The model under review builds one solid part; all positions refer to its coordinate system, in mm. Round coordinates to 2 decimals unless told otherwise and drop trailing zeros. Write each loop counter-clockwise with the first axis right and the second up, starting at its lowest first coordinate (ties: lowest second). Pieces come first, ordered by that corner, then holes. Notation, with made-up numbers: (-5.5, 23) - (49.5, 23) arc R29 cw to (49.5, 49) - close; hole circle Ø10 at (17.5, 83). An arc over 180 degrees is marked (long way). Return JSON: item names as keys, results as strings.
from build123d import *

# Parameters (mm, degrees)
EXTRUDE001_DEPTH = 3
FACE001_W        = 6
FACE001_H        = 15.392872
EXTRUDE002_DEPTH = 3
EXTRUDE003_DEPTH = 3
FACE003_W        = 15.392872
FACE003_H        = 6
EXTRUDE004_DEPTH = 3
EXTRUDE005_DEPTH = 3
EXTRUDE006_DEPTH = 3
EXTRUDE007_DEPTH = 3
FACE007_W        = 10
FACE007_H        = 10
EXTRUDE008_DEPTH = 3
EXTRUDE009_DEPTH = 3
EXTRUDE010_DEPTH = 3
EXTRUDE012_DEPTH = 3
FACE012_W        = 6
FACE012_H        = 15.392872
EXTRUDE013_DEPTH = 3
FACE010_W        = 15.392872
FACE010_H        = 6
EXTRUDE011_DEPTH = 3
EXTRUDE_DEPTH    = 1.5


with BuildPart() as extrude001:
    # Face → Extrude001 (new body)
    with BuildSketch(Plane(origin=(-12.399665, 12.399665, 0), x_dir=(0, 1, 0), z_dir=(0, 0, 1))):
        Polygon((4, -2), (-2, 4), (-2, -2), align=None)
    extrude(amount=EXTRUDE001_DEPTH)


with BuildPart() as extrude002:
    # Face001 → Extrude002 (new body)
    with BuildSketch(Plane(origin=(0, 13.399665, 0), x_dir=(0, 1, 0), z_dir=(0, 0, 1))):
        Rectangle(FACE001_W, FACE001_H)
    extrude(amount=EXTRUDE002_DEPTH)


with BuildPart() as extrude003:
    # Face002 → Extrude003 (new body)
    with BuildSketch(Plane(origin=(12.399665, 12.399665, 0), x_dir=(0, 1, 0), z_dir=(0, 0, 1))):
        Polygon((-2, -4), (4, 2), (-2, 2), align=None)
    extrude(amount=EXTRUDE003_DEPTH)


with BuildPart() as extrude004:
    # Face003 → Extrude004 (new body)
    with BuildSketch(Plane(origin=(13.399665, 0, 0), x_dir=(0, 1, 0), z_dir=(0, 0, 1))):
        Rectangle(FACE003_W, FACE003_H)
    extrude(amount=EXTRUDE004_DEPTH)


with BuildPart() as extrude005:
    # Face004 → Extrude005 (new body)
    with BuildSketch(Plane(origin=(12.399665, -12.399665, 0), x_dir=(0, 1, 0), z_dir=(0, 0, 1))):
        Polygon((2, -4), (2, 2), (-4, 2), align=None)
    extrude(amount=EXTRUDE005_DEPTH)


with BuildPart() as extrude006:
    # Face005 → Extrude006 (new body)
    with BuildSketch(Plane(origin=(7.712675, 0, 0), x_dir=(0, -1, 0), z_dir=(0, 0, -1))):
        Polygon((5.998742, 0.712675), (-5.998742, 0.712675), (-6.697694, -0.686991), (6.697694, -0.686991), align=None)
    extrude(amount=-EXTRUDE006_DEPTH)


with BuildPart() as extrude007:
    # Face006 → Extrude007 (new body)
    with BuildSketch(Plane(origin=(0, 7.712675, 0), x_dir=(0, -1, 0), z_dir=(0, 0, -1))):
        Polygon((-0.686991, 6.697694), (-0.686991, -6.697694), (0.712675, -5.998742), (0.712675, 5.998742), align=None)
    extrude(amount=-EXTRUDE007_DEPTH)


with BuildPart() as extrude008:
    # Face007 → Extrude008 (new body)
    with BuildSketch(Plane(origin=(0, 0, 0), x_dir=(0, 1, 0), z_dir=(0, 0, 1))):
        Rectangle(FACE007_W, FACE007_H)
    extrude(amount=EXTRUDE008_DEPTH)


with BuildPart() as extrude009:
    # Face008 → Extrude009 (new body)
    with BuildSketch(Plane(origin=(0, -7.712675, 0), x_dir=(0, -1, 0), z_dir=(0, 0, -1))):
        Polygon((-0.712675, 5.998742), (-0.712675, -5.998742), (0.686991, -6.697694), (0.686991, 6.697694), align=None)
    extrude(amount=-EXTRUDE009_DEPTH)


with BuildPart() as extrude010:
    # Face009 → Extrude010 (new body)
    with BuildSketch(Plane(origin=(-7.712675, 0, 0), x_dir=(0, -1, 0), z_dir=(0, 0, -1))):
        Polygon((6.697694, 0.686991), (-6.697694, 0.686991), (-5.998742, -0.712675), (5.998742, -0.712675), align=None)
    extrude(amount=-EXTRUDE010_DEPTH)


with BuildPart() as extrude012:
    # Face011 → Extrude012 (new body)
    with BuildSketch(Plane(origin=(-12.399665, -12.399665, 0), x_dir=(0, 1, 0), z_dir=(0, 0, 1))):
        Polygon((2, -2), (2, 4), (-4, -2), align=None)
    extrude(amount=EXTRUDE012_DEPTH)


with BuildPart() as extrude013:
    # Face012 → Extrude013 (new body)
    with BuildSketch(Plane(origin=(0, -13.399665, 0), x_dir=(0, 1, 0), z_dir=(0, 0, 1))):
        Rectangle(FACE012_W, FACE012_H)
    extrude(amount=EXTRUDE013_DEPTH)


with BuildPart() as extrude011:
    # Face010 → Extrude011 (new body)
    with BuildSketch(Plane(origin=(-13.399665, 0, 0), x_dir=(0, 1, 0), z_dir=(0, 0, 1))):
        Rectangle(FACE010_W, FACE010_H)
    extrude(amount=EXTRUDE011_DEPTH)


with BuildPart() as cut012:
    # Face013 → Extrude (new body)
    with BuildSketch(Plane(origin=(0, 0, 0), x_dir=(0, -1, 0), z_dir=(0, 0, -1))):
        with BuildLine():
            ThreePointArc((23.399665, 8.800889), (14.849242, 14.849242), (8.800889, 23.399665))
            Line((8.800889, 23.399665), (-8.800889, 23.399665))
            ThreePointArc((-8.800889, 23.399665), (-14.849242, 14.849242), (-23.399665, 8.800889))
            Line((-23.399665, 8.800889), (-23.399665, -8.800889))
            ThreePointArc((-23.399665, -8.800889), (-14.849242, -14.849242), (-8.800889, -23.399665))
            Line((-8.800889, -23.399665), (8.800889, -23.399665))
            ThreePointArc((8.800889, -23.399665), (14.849242, -14.849242), (23.399665, -8.800889))
            Line((23.399665, -8.800889), (23.399665, 8.800889))
        make_face()
    extrude(amount=-EXTRUDE_DEPTH)

    # Cut: cut Extrude011
    add(extrude011.part, mode=Mode.SUBTRACT)

    # Cut001: cut Extrude013
    add(extrude013.part, mode=Mode.SUBTRACT)

    # Cut002: cut Extrude012
    add(extrude012.part, mode=Mode.SUBTRACT)

    # Cut003: cut Extrude010
    add(extrude010.part, mode=Mode.SUBTRACT)

    # Cut004: cut Extrude009
    add(extrude009.part, mode=Mode.SUBTRACT)

    # Cut005: cut Extrude008
    add(extrude008.part, mode=Mode.SUBTRACT)

    # Cut006: cut Extrude007
    add(extrude007.part, mode=Mode.SUBTRACT)

    # Cut007: cut Extrude006
    add(extrude006.part, mode=Mode.SUBTRACT)

    # Cut008: cut Extrude005
    add(extrude005.part, mode=Mode.SUBTRACT)

    # Cut009: cut Extrude004
    add(extrude004.part, mode=Mode.SUBTRACT)

    # Cut010: cut Extrude003
    add(extrude003.part, mode=Mode.SUBTRACT)

    # Cut011: cut Extrude002
    add(extrude002.part, mode=Mode.SUBTRACT)

    # Cut012: cut Extrude001
    add(extrude001.part, mode=Mode.SUBTRACT)


solid = cut012.part
(1) Mouldability with a two-part tool opening along X and no side actions: class faces 1 (the cylindrical face through (14.7, 15, 0.7)), 2 (the flat face through (0, -10, 0)), 3 (the flat face through (13, 10.4, 1)) as released by +X, released by -X, zero draft, split by the parting line, or undercut.
Filled in:
{"face 1": "released by +X", "face 2": "zero draft", "face 3": "undercut"}
(2) Wall thickness on line 1 (Y direction, x = -5.5, z = 0.2); line 2 (X direction, y = 1, z = 0.15): over which ranges is each line inside the solid? List them lowest first.
Filled in:
{"line 1": "y = -23.4 to -16.4, -10.4 to -8.4, -7 to 7, 8.4 to 10.4, 16.4 to 23.4", "line 2": "x = -23.4 to -16.4, -10.4 to -8.4, -7 to -5, 5 to 7, 8.4 to 10.4, 16.4 to 23.4"}
(3) Add section D-D (z = 1). Give the number of separate pieces and of enclosed holes in the cut face, plus the area to 3 significant figures.
Filled in:
{"separate pieces": "1", "enclosed holes": "13", "area": "1,050 mm2"}
(4) Add section B-B (x = -13.5). Write out the cut boundary in (y, z), plus the area to 3 significant figures.
Filled in:
{"outline": "(-16.29, 0) - (-13.3, 0) - (-13.3, 1.5) - (-16.29, 1.5) - close; (-10.4, 0) - (-7.7, 0) - (-7.7, 1.5) - (-10.4, 1.5) - close; (7.7, 0) - (10.4, 0) - (10.4, 1.5) - (7.7, 1.5) - close; (13.3, 0) - (16.29, 0) - (16.29, 1.5) - (13.3, 1.5) - close", "area": "17.1 mm2"}
(5) Add section A-A (y = -2). Write out the cut boundary in (x, z), plus the area to 3 significant figures.
Filled in:
{"outline": "(-23.4, 0) - (-16.4, 0) - (-16.4, 1.5) - (-23.4, 1.5) - close; (-10.4, 0) - (-8.4, 0) - (-8.4, 1.5) - (-10.4, 1.5) - close; (-7, 0) - (-5, 0) - (-5, 1.5) - (-7, 1.5) - close; (5, 0) - (7, 0) - (7, 1.5) - (5, 1.5) - close; (8.4, 0) - (10.4, 0) - (10.4, 1.5) - (8.4, 1.5) - close; (16.4, 0) - (23.4, 0) - (23.4, 1.5) - (16.4, 1.5) - close", "area": "33.0 mm2"}
(6) Clearance check with flat-ended pins moving along their axes: pin 1 Ø0.8 at (y, z) = (13.5, 1) entering from -X; pin 2 Ø0.8 at (y, z) = (13, 1) entering from +X. State where each tip first meets the part, or that it passes through.
Filled in:
{"pin 1": "stops at x = -16.75", "pin 2": "stops at x = 17.36"}
(7) Add section C-C (y = -13). Write out the cut boundary in (x, z), plus the area to 3 significant figures.
Filled in:
{"outline": "(-16.87, 0) - (-13.8, 0) - (-13.8, 1.5) - (-16.87, 1.5) - close; (-10.4, 0) - (-7.7, 0) - (-7.7, 1.5) - (-10.4, 1.5) - close; (7.7, 0) - (10.4, 0) - (10.4, 1.5) - (7.7, 1.5) - close; (13.8, 0) - (16.87, 0) - (16.87, 1.5) - (13.8, 1.5) - close", "area": "17.3 mm2"}
